```python
from build123d import *

# Parameters (mm, degrees)
SKETCH13_R              = 4.6
SKETCH13_W              = 80
SKETCH13_H              = 55
BOSS_EXTRUDE4_DEPTH     = 15
CUT_EXTRUDE1_DEPTH      = 9
CUT_EXTRUDE2_DEPTH      = 146.691454794
CUT_EXTRUDE2_DEPTH_BACK = 6
SKETCH16_R              = 1.75
FILLET1_R               = 2
SKETCH17_R              = 1.75
CUT_EXTRUDE3_DEPTH      = 10
SKETCH18_R              = 1.75
SKETCH18_R_2            = 1.9
CUT_EXTRUDE4_DEPTH      = 10
SKETCH21_R              = 4.6
SKETCH21_R_2            = 3.1
BOSS_EXTRUDE7_DEPTH     = 2
SKETCH22_R              = 3.1
CUT_EXTRUDE5_DEPTH      = 1.5
SKETCH23_W              = 9
SKETCH23_H              = 7
SKETCH23_R              = 1.75
BOSS_EXTRUDE8_DEPTH     = 3


with BuildPart() as part:
    # Sketch13 → Boss-Extrude4 (new body)
    with BuildSketch(Plane(origin=(0, 0, 0), x_dir=(0, 0, -1), z_dir=(1, 0, 0))):
        Polygon((0, 0), (-24, 10), (-24, 65), (0, 75), (10, 75), (10, 65), (90, 65), (90, 75), (100, 75), (124, 65), (124, 10), (100, 0), align=None)
        with Locations((-10.8, 31)):
            Circle(SKETCH13_R, mode=Mode.SUBTRACT)
        with Locations((110.8, 31)):
            Circle(SKETCH13_R, mode=Mode.SUBTRACT)
        with Locations((50, 32.5)):
            Rectangle(SKETCH13_W, SKETCH13_H, mode=Mode.SUBTRACT)
    extrude(amount=BOSS_EXTRUDE4_DEPTH)

    # Sketch14 → Cut-Extrude1 (cut)
    with BuildSketch(Plane(origin=(15, 0, 0), x_dir=(0, 0, -1), z_dir=(1, 0, 0))):
        Polygon((10, 70.5), (10, 60.5), (90, 60.5), (90, 70.5), (90, 75), (92, 75), (92, 70), (99, 70), (119, 61.666666667), (119, 13.333333333), (99, 5), (1, 5), (-19, 13.333333333), (-19, 61.666666667), (1, 70), (8, 70), (8, 75), (10, 75), align=None)
    extrude(amount=-CUT_EXTRUDE1_DEPTH, mode=Mode.SUBTRACT)

    # Sketch16 → Cut-Extrude2 (cut, two sides: drawn at the far end of the back side and taken through both)
    with BuildSketch(Plane(origin=(0, 75, 0), x_dir=(1, 0, 0), z_dir=(0, 1, 0)).offset(-CUT_EXTRUDE2_DEPTH_BACK)):
        with Locations(Location((10, 4, 0), (0, 0, 90))):
            Circle(SKETCH16_R)
        with Locations(Location((10, 96, 0), (0, 0, 90))):
            Circle(SKETCH16_R)
    extrude(amount=CUT_EXTRUDE2_DEPTH + CUT_EXTRUDE2_DEPTH_BACK, mode=Mode.SUBTRACT)

    # Fillet1
    fillet1_edges = [part.edges().sort_by_distance(p)[0] for p in [
        (6, 62.75, -90),
        (6, 62.75, -10),
        (15, 62.75, -90),
        (15, 62.75, -10),
    ]]
    fillet(fillet1_edges, radius=FILLET1_R)

    # Sketch17 → Cut-Extrude3 (cut)
    with BuildSketch(Plane(origin=(0, 65, 0), x_dir=(1, 0, 0), z_dir=(0, 1, 0))):
        with Locations(Location((10, 15, 0), (0, 0, 270))):
            Circle(SKETCH17_R)
        with Locations(Location((10, 85, 0), (0, 0, 270))):
            Circle(SKETCH17_R)
        with Locations(Location((10, 72, 0), (0, 0, 270))):
            Circle(SKETCH17_R)
        with Locations(Location((10, 28, 0), (0, 0, 270))):
            Circle(SKETCH17_R)
    extrude(amount=-CUT_EXTRUDE3_DEPTH, mode=Mode.SUBTRACT)

    # Sketch18 → Cut-Extrude4 (cut)
    with BuildSketch(Plane.XZ):
        with Locations(Location((9, -20, 0), (0, 0, 270))):
            Circle(SKETCH18_R)
        with Locations(Location((9, -80, 0), (0, 0, 270))):
            Circle(SKETCH18_R)
        with Locations(Location((9, -30.5, 0), (0, 0, 270))):
            Circle(SKETCH18_R_2)
        with Locations(Location((9, -69.5, 0), (0, 0, 270))):
            Circle(SKETCH18_R_2)
    extrude(amount=-CUT_EXTRUDE4_DEPTH, mode=Mode.SUBTRACT)

    # Sketch21 → Boss-Extrude7 (add)
    # profile 1 of 2: a face of its own
    with BuildSketch(Plane.ZY):
        with Locations((-110.8, 31)):
            Circle(SKETCH21_R)
        with Locations((-110.8, 31)):
            Circle(SKETCH21_R_2, mode=Mode.SUBTRACT)
    # profile 2 of 2: a face of its own
    with BuildSketch(Plane.ZY):
        with Locations((10.8, 31)):
            Circle(SKETCH21_R)
        with Locations((10.8, 31)):
            Circle(SKETCH21_R_2, mode=Mode.SUBTRACT)
    extrude(amount=-BOSS_EXTRUDE7_DEPTH)

    # Sketch22 → Cut-Extrude5 (cut)
    with BuildSketch(Plane(origin=(0, 5, 0), x_dir=(1, 0, 0), z_dir=(0, 1, 0))):
        with Locations(Location((9, 20, 0), (0, 0, 270))):
            Circle(SKETCH22_R)
        with Locations(Location((9, 80, 0), (0, 0, 270))):
            Circle(SKETCH22_R)
    extrude(amount=-CUT_EXTRUDE5_DEPTH, mode=Mode.SUBTRACT)

    # Sketch23 → Boss-Extrude8 (add)
    # profile 1 of 2: a face of its own
    with BuildSketch(Plane.XZ.offset(-70)):
        with Locations((10.5, -95.5)):
            Rectangle(SKETCH23_W, SKETCH23_H)
        with Locations(Location((10, -96, 0), (0, 0, 270))):
            Circle(SKETCH23_R, mode=Mode.SUBTRACT)
    # profile 2 of 2: a face of its own
    with BuildSketch(Plane.XZ.offset(-70)):
        with Locations((10.5, -4.5)):
            Rectangle(SKETCH23_W, SKETCH23_H)
        with Locations(Location((10, -4, 0), (0, 0, 270))):
            Circle(SKETCH23_R, mode=Mode.SUBTRACT)
    extrude(amount=BOSS_EXTRUDE8_DEPTH)


solid = part.part
```
The model under review builds one solid part; all positions refer to its coordinate system, in mm. A direction names the side the tool comes from. Round coordinates to 2 decimals unless told otherwise and drop trailing zeros. Loops run counter-clockwise (first coordinate to the right, second up) from the corner with the lowest first, then second, coordinate; pieces in that order, holes last.
Item 1: For faces 4 (the face through (10.56, 65.89, -108.86)), 5 (the face through (9.1, 4.3, -23.1)), 6 (the face through (3, 70, -10)), list the 3-axis set-ups (+Z, -Z, +X, -X, +Y, -Y) from which the entire face can be reached by the end or side of a thin tool; tool diameter is ignored.
Determined:
face 4: +X
face 5: none
face 6: +X, -X, +Y
Item 2: Take a section at C-C (z = -80). Write out the cut boundary in (x, y).
Determined:
outline: (0, 0) - (7.25, 0) - (7.25, 3.5) - (5.9, 3.5) - (5.9, 5) - (0, 5) - close; (0, 60) - (6, 60) - (6, 60.5) - (15, 60.5) - (15, 65) - (0, 65) - close; (10.75, 0) - (15, 0) - (15, 5) - (12.1, 5) - (12.1, 3.5) - (10.75, 3.5) - close
Item 3: Clearance check with flat-ended pins moving along their axes: pin 1 Ø5 at (y, z) = (44, -87) entering from -X; pin 2 Ø0.9 at (x, y) = (10, 69) entering from +Z; pin 3 Ø4 at (x, z) = (10, -72) entering from +Y; pin 4 Ø9 at (x, y) = (9.5, 71) entering from -Z. State where each tip first meets the part, or that it passes through.
Determined:
pin 1: passes through
pin 2: stops at z = 15.48
pin 3: stops at y = 65
pin 4: stops at z = -120.4
Item 4: For line 1 (Z direction, x = 4, y = 31); line 2 (Z direction, x = 12, y = 50); line 3 (Y direction, x = 8.5, z = -50.5), list the stretches that pass through material, from the lowest coordinate up.
Determined:
line 1: z = -124 to -115.4, -106.2 to -90, -10 to 6.2, 15.4 to 24
line 2: z = -124 to -119, 19 to 24
line 3: y = 0 to 5, 60.5 to 65
Item 5: Take a section at D-D (z = 10.8). Write out the cut boundary in (x, y), then the cut area to 3 significant figures.
Determined:
outline: (0, 4.5) - (15, 4.5) - (15, 9.92) - (6, 9.92) - (6, 26.4) - (2, 26.4) - (2, 27.9) - (0, 27.9) - close; (0, 34.1) - (2, 34.1) - (2, 35.6) - (6, 35.6) - (6, 65.08) - (15, 65.08) - (15, 70.5) - (0, 70.5) - close
area: 444 mm2
Item 6: Mouldability with a two-part tool opening along Y and no side actions: class faces 1 (the face through (10.526, 62.782, -83.331)), 2 (the face through (7, 5, -49)), 3 (the face through (7, 70, 12)) as released by +Y, released by -Y, zero draft, split by the parting line, or undercut.
Determined:
face 1: zero draft
face 2: undercut
face 3: released by +Y
Item 7: Take a section at B-B (z = -96). Write out the cut boundary in (x, y).
Determined:
outline: (0, 0) - (15, 0) - (15, 5) - (6, 5) - (6, 67) - (8.25, 67) - (8.25, 75) - (0, 75) - close; (11.75, 67) - (15, 67) - (15, 75) - (11.75, 75) - close
Item 8: Take a section at A-A (y = 56). Write out the cut boundary in (x, z).
Determined:
outline: (0, -124) - (15, -124) - (15, -119) - (6, -119) - (6, -90) - (0, -90) - close; (0, -10) - (6, -10) - (6, 19) - (15, 19) - (15, 24) - (0, 24) - close
